Read the model definition and answer for the solid it produces. Units are mm, in the model's axes. A direction names the side the tool comes from. Coordinates: 2 decimals unless noted, no trailing zeros. Order: outer loops, then holes, each group sorted by start corner. A loop starts at its lowest first (then second) coordinate and runs counter-clockwise, first axis right, second up. Notation, with made-up numbers: (25, -37) -> (50, -37) arc R24 cw to (50, 2) -> close; hole circle Ø9 at (24, 56.25). An arc over 180 degrees is marked (long way). Answer as a JSON object with one key per item and string values. Group by question number.
1) A tool of negligible diameter and unlimited length cuts with its end or side. For faces 5 (the flat face through (-1.5, -12.5, 4.3)), 6 (the flat face through (0, -6, -6.5)), 7 (the flat face through (0, -13, 4.73)), from which of +Z, -Z, +X, -X, +Y, -Y can it reach the whole face along a straight path? Write none if from no direction.
2) Given pin 1 (3.5 mm diameter, centred on x = 0, y = -13, fed in from -Z); pin 2 (3 mm diameter, centred on y = -10.5, z = 4.5, fed in from +X); pin 3 (0.6 mm diameter, centred on y = -11.5, z = -5, fed in from +X); pin 4 (2.5 mm diameter, centred on x = 1, z = 1, fed in from -Y), each flat-ended and moving along its own axis, determine where each tip first touches the part or whether it passes through.
3) Consider L1, parallel to X at y = 2, z = 0; L2, parallel to Y at x = 3, z = 1.5; L3, parallel to Y at x = -1.75, z = 5.25. Determine where each line is inside the solid, lowest interval first.
4) Determine the mould class of faces 1 (the flat face through (0, -10.3, -1)), 2 (the flat face through (0, -6, 6.5)), 3 (the flat face through (0, -14.8, 4.3)), 4 (the cylindrical face through (0.062, 11.283, -1.386)) for opening direction Z: released by +Z, released by -Z, zero draft, split by the parting line, or undercut.
5) Section A-A on y = 2.5 is taken. Determine the outline of the cut face in (x, z), and give its area (3 significant figures).
6) Section D-D on x = 3.5 is taken. Determine the outline of the cut face in (y, z), and give its area (3 significant figures).
7) Section B-B on z = 3.5 is taken. Determine the outline of the cut face in (x, y).
from build123d import *

# Parameters (mm, degrees)
SKETCH1_R           = 3.16357
SKETCH1_R_2         = 2.56357
BOSS_EXTRUDE1_DEPTH = 8
SKETCH2_R           = 4
BOSS_EXTRUDE2_DEPTH = 0.9
SKETCH3_W           = 7.9
SKETCH3_H           = 13
BOSS_EXTRUDE3_DEPTH = 9.4
SKETCH4_W           = 3
SKETCH4_H           = 0.8
BOSS_EXTRUDE4_DEPTH = 4.5


with BuildPart() as part:
    # Sketch1 → Boss-Extrude1 (new body)
    with BuildSketch(Plane(origin=(0, 0, 0), x_dir=(1, 0, 0), z_dir=(0, 1, 0))):
        with Locations(Location((0, 0, 0), (0, 0, 270))):
            Circle(SKETCH1_R)
        with Locations(Location((0, 0, 0), (0, 0, 270))):
            Circle(SKETCH1_R_2, mode=Mode.SUBTRACT)
    extrude(amount=BOSS_EXTRUDE1_DEPTH)

    # Sketch2 → Boss-Extrude2 (add)
    with BuildSketch(Plane.XZ):
        with Locations(Location((0, 0, 0), (0, 0, 270))):
            Circle(SKETCH2_R)
    extrude(amount=BOSS_EXTRUDE2_DEPTH)

    # Sketch3 → Boss-Extrude3 (add)
    with BuildSketch(Plane.XZ.offset(0.9)):
        Rectangle(SKETCH3_W, SKETCH3_H)
    extrude(amount=BOSS_EXTRUDE3_DEPTH)

    # Sketch4 → Boss-Extrude4 (add)
    with BuildSketch(Plane.XZ.offset(10.3)):
        with Locations((0, 4.330352395)):
            Rectangle(SKETCH4_W, SKETCH4_H)
        Rectangle(SKETCH4_W, SKETCH4_H)
        with Locations((0, -4.801802051)):
            Rectangle(SKETCH4_W, SKETCH4_H)
    extrude(amount=BOSS_EXTRUDE4_DEPTH)

    # Sketch5 → Revolve1 (revolve)
    with BuildSketch(Plane(origin=(0, 0, 0), x_dir=(0, 0, -1), z_dir=(1, 0, 0)), mode=Mode.PRIVATE) as revolve1_sk:
        with BuildLine():
            Line((4.373491762, 17.691665566), (-1.520701627, 5.051527053))
            Line((-1.520701627, 5.051527053), (-0.251870725, 4.459861486))
            Line((-0.251870725, 4.459861486), (6.23398823, 18.368830902))
            ThreePointArc((6.23398823, 18.368830902), (5.163494463, 18.415569669), (4.373491762, 17.691665566))
        make_face()
    revolve(revolve1_sk.sketch.rotate(Axis((0, 15.555621566, -4.922167173), (0, -0.9063077870366496, 0.4226182617407002)), 180), axis=Axis((0, 15.555621566, -4.922167173), (0, -0.9063077870366496, 0.4226182617407002)))


solid = part.part
Worked answers:
{
 "1": {"face 5": "+Z, -Z, -X, -Y", "face 6": "-Z, +X, -X, -Y", "face 7": "+Z, +X, -X, -Y"},
 "2": {"pin 1": "stops at z = -5.2", "pin 2": "stops at x = 3.95", "pin 3": "stops at x = 1.5", "pin 4": "stops at y = -14.8"},
 "3": {"L1": "x = -3.16 to -2.56, 2.56 to 3.16", "L2": "y = -10.3 to 0", "L3": "y = -10.3 to -0.9"},
 "4": {"face 1": "undercut", "face 2": "released by +Z", "face 3": "zero draft", "face 4": "undercut"},
 "5": {"outline": "circle Ø6.33 at (0, 0); hole circle Ø5.13 at (0, 0)", "area": "10.8 mm²"},
 "6": {"outline": "(-10.3, -6.5) -> (-0.9, -6.5) -> (-0.9, -1.94) -> (0, -1.94) -> (0, 1.94) -> (-0.9, 1.94) -> (-0.9, 6.5) -> (-10.3, 6.5) -> close", "area": "126 mm²"},
 "7": {"outline": "(-3.95, -10.3) -> (3.95, -10.3) -> (3.95, -0.9) -> (1.94, -0.9) -> (1.94, 0) -> (-1.94, 0) -> (-1.94, -0.9) -> (-3.95, -0.9) -> close"}
}
